Autodesk Inventor part; units mm, degrees
ref_plane "Work Plane1" through (17.8247, 6.5, -8.1364) normal (0, 0, 1) x (1, 0, 0)
ref_plane "Work Plane5" through (0, 6, 0) normal (0, 1, 0) x (1, 0, 0)
ref_plane "Work Plane6" through (-2.6753, 0, 1.9193) normal (-1, 0, 0) x (0, 0, 1)
sketch "Sketch1" plane through (0, 0, 0) normal (0, 1, 0) x (-1, 0, 0)
  line L0 (16.1753, 16.3636) -> (-28.8247, 16.3636)
  line L1 (-28.8247, 16.3636) -> (-28.8247, 6.3636)
  line L2 (16.1753, 6.3636) -> (16.1753, 16.3636)
  line L3 (-17.8247, 6.3636) -> (-17.8247, 1.3636)
  line L4 (-17.8247, 1.3636) -> (5.1753, 1.3636)
  line L5 (5.1753, 1.3636) -> (5.1753, 6.3636)
  line L6 (-28.8247, 6.3636) -> (-17.8247, 6.3636)
  line L7 (5.1753, 6.3636) -> (16.1753, 6.3636)
  point P0 (0, 0)
  dimension "d4" = 45
  dimension "d5" = 5
  dimension "d6" = 5
  dimension "d7" = 11
  dimension "d8" = 11
  dimension "d9" = 23
  dimension "d10" = 10
extrude "Extrusion1" add sketch "Sketch1" along normal blind 6
sketch "Sketch4" plane through (17.8247, 0, 6.3636) normal (1, 0, 0) x (0, 0, -1)
  circle A0 centre (8, 6.5) radius 6.5
  line L0 (0, 6) -> (5, 6)
  line L1 (0, 0) -> (0, 6)
  line L2 (0, 0) -> (5, 0)
  line L3 (5, 0) -> (16.9814, 0)
  point P0 (6.3636, 0)
  dimension "d20" = 13
  dimension "d36" = 8
extrude "Extrusion4" add sketch "Sketch4" against normal up to surface (23 mm away) contours A0
fillet "Fillet1" radius 12 2 edges at (6.3247, 0.7337, 1.3636) (6.3247, 0, 1.3636)
sketch "Sketch5" plane through (17.8247, 0, 6.3636) normal (1, 0, 0) x (0, 0, -1)
  circle A0 centre (8, 6.5) radius 6.5
  circle A1 centre (8, 6.5) radius 2.5
  point P0 (6.3636, 0)
  point P1 (1.5193, 6)
  point P2 (7.416, 0.0263)
  dimension "d27" = 5
extrude "Extrusion5" cut sketch "Sketch5" against normal through all contours A1
ref_plane "Work Plane1" through (17.8247, 6.5, -8.1364) normal (0, 0, 1) x (1, 0, 0)
sketch "Sketch6" plane through (0, 6, 0) normal (0, 1, 0) x (1, 0, 0)
  circle A0 centre (-9.0753, -9.6636) radius 2.5
  circle A1 centre (21.7247, -9.6636) radius 2.5
  line L0 (37.8247, 8.1364) -> (-25.1753, 8.1364)
  line L1 (28.8247, -16.3636) -> (28.8247, -6.3636)
  line L2 (-16.1753, -6.3636) -> (-16.1753, -16.3636)
  point P0 (0, 0)
  dimension "d33" = 5
  dimension "d34" = 5
  dimension "d35" = 17.8
  dimension "d37" = 17.8
  dimension "d38" = 7.1
  dimension "d39" = 30.8
  dimension "d40" = 7.1
extrude "Extrusion6" cut sketch "Sketch6" against normal through all
move faces "Move1" translate (-2.5, 0, 0) faces at (17.8247, 2, 4.3758)
move faces "Move2" translate (2.5, 0, 0) faces at (-5.1753, 2, 4.3758) (8.4913, 6.099, -4.104)
sketch "Sketch7" plane through (0, 6, 0) normal (0, 1, 0) x (1, 0, 0)
  line L0 (-2.6753, -4.8444) -> (-2.6753, -6.3636)
  line L1 (-2.6753, -4.8444) -> (-2.6753, -14.145)
  line L2 (15.3247, -6.3636) -> (15.3247, -1.9193)
  line L3 (15.3247, -4.1415) -> (-2.6753, -4.1415)
  line L4 (-2.6753, -4.1415) -> (-2.6753, -15.1415)
  line L5 (-2.6753, -15.1415) -> (15.3247, -15.1415)
  line L6 (15.3247, -15.1415) -> (15.3247, -4.1415)
  point P0 (0, 0)
  dimension "d52" = 18
  dimension "d53" = 11
extrude "Extrusion7" add sketch "Sketch7" along normal blind 2
fillet "Fillet2" radius 2 1 edges at (6.3247, 8, 4.6882)
ref_plane "Work Plane5" through (0, 6, 0) normal (0, 1, 0) x (1, 0, 0)
sketch "Sketch8" plane through (0, 6, 0) normal (0, 1, 0) x (1, 0, 0)
  line L0 (-2.6753, -0.8636) -> (-2.6753, 4.1364)
  line L1 (-2.6753, -15.1415) -> (15.3247, -15.1415)
  line L2 (-2.6753, 0) -> (15.3247, 0)
  line L3 (15.3247, 0) -> (15.3247, -15.1415)
  line L4 (15.3247, -15.1415) -> (-2.6753, -15.1415)
  line L5 (-2.6753, -15.1415) -> (-2.6753, 0)
  point P0 (0, 0)
extrude "Extrusion8" cut sketch "Sketch8" along normal blind 0.5
ref_plane "Work Plane6" through (-2.6753, 0, 1.9193) normal (-1, 0, 0) x (0, 0, 1)
sketch "Sketch10" plane through (-2.6753, 0, 1.9193) normal (-1, 0, 0) x (0, 0, 1)
  line L0 (-1.0557, 6.5) -> (13.2222, 6.5)
  line L1 (13.2222, 6.5) -> (13.2222, 8)
  line L2 (4.1903, 8) -> (13.2222, 8)
  arc A0 (2.3677, 9.1765) -> (-2.9717, 0.0263) centre (-3.5557, 6.5) ccw
  arc A1 (-0.9468, 0.0374) -> (-2.9717, 0.0263) centre (-1.8936, -11.9252) ccw
  arc A2 (-0.9468, 0.0374) -> (0, 0) centre (0, 12) ccw
  line L3 (0, 0) -> (4.4443, 0)
  line L4 (4.4443, 0) -> (4.4443, 6)
  line L5 (4.4443, 6) -> (-1.1062, 6)
  arc A3 (-1.0557, 6.5) -> (-1.1062, 6) centre (-3.5557, 6.5) ccw
  arc A4 (2.3677, 9.1765) -> (4.1903, 8) centre (4.1903, 10) ccw
  point P0 (-1.9193, 0)
extrude "Extrusion9" add sketch "Sketch10" along normal up to surface (13.5 mm away)
sketch "Sketch11" plane through (-2.6753, 0, 1.9193) normal (-1, 0, 0) x (0, 0, 1)
  line L0 (2.7662, 9.2202) -> (17.7662, 9.2202)
  line L1 (17.7662, 9.2202) -> (17.7662, 6.2202)
  line L2 (17.7662, 6.2202) -> (2.7662, 6.2202)
  line L3 (2.7662, 6.2202) -> (2.7662, 9.2202)
  point P0 (-1.9193, 0)
  point P1 (-3.5557, 6.5)
  dimension "d82" = 15
  dimension "d83" = 3
sketch "Sketch12" plane through (15.3247, 0, 6.3636) normal (1, 0, 0) x (0, 0, -1)
  arc A0 (3.5, 6.5) -> (3.5, 6.5) centre (8, 6.5) ccw
  line L0 (3.5, 6.5) -> (3.5, 6.5)
  circle A1 centre (8, 6.5) radius 2.5
  circle A2 centre (8, 6.5) radius 4.5
  point P0 (6.3636, 0)
  dimension "d72" = 2
sketch "Sketch13" plane through (0, 8, 0) normal (0, 1, 0) x (1, 0, 0)
  line L0 (15.3247, -6.4035) -> (-2.6753, -6.4035)
  line L1 (15.3247, -15.1415) -> (15.3247, -0.8636)
  line L2 (-2.6753, -14.1415) -> (-2.6753, -2.35)
  circle A0 centre (6.3247, -10.8459) radius 2.5
  point P0 (0, 0)
  point P1 (15.3247, -3.7322)
  dimension "d68" = 5
extrude "Extrusion12" cut sketch "Sketch13" against normal through all
extrude "Extrusion13" cut sketch "Sketch12" against normal through all
extrude "Extrusion15" cut sketch "Sketch11" along normal up to surface (13.5 mm away)
ref_plane "Work Plane7" through (0, 0, 0) normal (0, 1, 0) x (1, 0, 0)
sketch "Sketch14" plane through (0, 0, 0) normal (0, 1, 0) x (1, 0, 0)
  circle A0 centre (6.3247, -10.8459) radius 2.5
  line L0 (10.0747, -8.6808) -> (10.0747, -13.0109)
  line L1 (10.0747, -13.0109) -> (6.3247, -15.176)
  line L2 (6.3247, -15.176) -> (2.5747, -13.0109)
  line L3 (2.5747, -13.0109) -> (2.5747, -8.6808)
  line L4 (2.5747, -8.6808) -> (6.3247, -6.5157)
  line L5 (6.3247, -6.5157) -> (10.0747, -8.6808)
  line L6 (15.3247, -15.1415) -> (15.3247, -6.1096)
  point P0 (0, 0)
  dimension "d89" = 7.5
extrude "Extrusion16" cut sketch "Sketch14" along normal blind 3.15
properties part number "Cerniera 3"
Check sheet for the modelled part. Datum: model origin and axes. Units: mm. A direction names the side the tool comes from. Round coordinates to 2 decimals unless told otherwise and drop trailing zeros. Order: outer loops, then holes, each group sorted by start corner. A loop starts at its lowest first (then second) coordinate and runs counter-clockwise, first axis right, second up.
(1) Cross-section at D-D, the plane y = 1.25. Enter the section's corners in (x, z), and give its area (3 significant figures).
(2) Go/stop test with flat-tipped pins: P1, Ø1.5, axis at x = 18, z = 8, coming from the +Y side; P2, Ø6, axis at x = 6.32, z = 10.85, coming from the -Y side; P3, Ø2, axis at x = -1.5, y = 4.5, coming from the -Z side; P4, Ø4, axis at y = 5.5, z = -1.5, coming from the +X side. Record where each tip stops, or that it passes through.
(3) Cross-section at C-C, the plane x = -8. Enter the section's corners in (y, z).
(4) Cross-section at A-A, the plane y = 5.5. Enter the section's corners in (x, z), and give its area (3 significant figures).
(5) Cross-section at B-B, the plane z = -4.25. Enter the section's corners in (x, y), and give its area (3 significant figures).
(6) Access from +Z, -Z, +X, -X, +Y, -Y to the whole of each face (thin tool, end or side, straight path). Record for faces 5 (the flat face through (15.325, 5, 3)), 6 (the flat face through (4.423, 1.553, 7.613)), 7 (the flat face through (6, 7, 15.142)), 8 (the flat face through (7, 6.5, 8)).
(7) Scan lines: probe 1 along Y at (x, z) = (6, 14.5); probe 2 along Z at (x, y) = (8, 3); probe 3 along X at (y, z) = (0.5, 4.25). Record each from-to range of solid material in increasing order.
(8) Draft check along Z on faces 1 (the cylindrical face through (6.45, 8.31, 5.04)), 2 (the flat face through (4, 8, 13)), 3 (the cylindrical face through (6.45, 9.6, -7.35)), 4 (the flat face through (8.2, 1.6, 7.6)). Enter one of: pulls with the +Z half, pulls with the -Z half, needs draft (parallel to the pull), parting line crosses it, or undercut.
Check sheet entries:
1. outline: (-16.18, -5.47) - (15.32, -5.47) - (15.32, 6.36) - (28.82, 6.36) - (28.82, 16.36) - (-16.18, 16.36) - close; hole circle Ø5 at (-9.08, 9.66); hole (2.57, 8.68) - (6.32, 6.52) - (10.07, 8.68) - (10.07, 13.01) - (6.32, 15.18) - (2.57, 13.01) - close; hole circle Ø5 at (21.72, 9.66)
1. area: 735 mm2
2. P1: stops at y = 6
2. P2: stops at y = 3.15
2. P3: stops at z = -8.06
2. P4: passes through
3. outline: (0, 1.92) arc R11.99 ccw to (0.04, 0.97) arc R12 cw to (0.03, -1.05) arc R6.5 ccw (long way) to (9.18, 4.29) arc R2 cw to (8.6, 4.69) - (6.5, 4.69) - (6.5, 2.86) arc R4.5 cw (long way) to (6, 2.84) - (6, 7.41) - (0, 7.41) - close; (0, 11.92) - (6, 11.92) - (6, 16.36) - (0, 16.36) - close
4. outline: (-16.18, -8.06) - (15.32, -8.06) - (15.32, -6.02) - (-16.18, -6.02) - close; (-16.18, 2.75) - (15.32, 2.75) - (15.32, 6.36) - (28.82, 6.36) - (28.82, 16.36) - (-16.18, 16.36) - close; hole circle Ø5 at (-9.08, 9.66); hole circle Ø5 at (6.32, 10.85); hole circle Ø5 at (21.72, 9.66)
4. area: 569 mm2
5. outline: (-16.18, 0.55) - (15.32, 0.55) - (15.32, 2.84) - (-16.18, 2.84) - close; (-16.18, 10.16) - (15.32, 10.16) - (15.32, 12.45) - (-16.18, 12.45) - close
5. area: 144 mm2
6. face 5: -Z, +X, +Y
6. face 6: -Y
6. face 7: +Z, +X, -X, +Y
6. face 8: +Z, +X, -X
7. probe 1: y = 3.15 to 6, 6.5 to 8
7. probe 2: z = -7.11 to -4.46, 1.19 to 7.48, 14.21 to 16.36
7. probe 3: x = -16.18 to 15.32
8. face 1: pulls with the +Z half
8. face 2: needs draft
8. face 3: parting line crosses it
8. face 4: undercut
